from build123d import *

# Parameters (mm, degrees)
F0_W     = 127
F0_H     = 127
F1_DEPTH = 12.7
F3_D     = 15.24
F3_DEPTH = 12.7
F5_D     = 6.35
F5_DEPTH = 12.7


with BuildPart() as f1:
    # F0 (on Top) → F1 (new body)
    with BuildSketch(Plane.XY):
        with Locations((10.277962, -0.006821)):
            Rectangle(F0_W, F0_H)
    extrude(amount=F1_DEPTH)

    # F3
    with Locations(Plane.XY.offset(12.7)):
        with Locations((-40.522038, 50.793179), (-40.522038, 0), (-40.522038, -50.806821)):
            Hole(F3_D / 2, depth=F3_DEPTH)

    # F5
    with Locations(Plane.XY.offset(12.7)):
        with Locations((64.830244, -38.106821), (64.830244, 50.793179), (64.830244, 38.093179), (64.830244, -50.806821)):
            Hole(F5_D / 2, depth=F5_DEPTH)


solid = f1.part
Model file for the job. Use its own axes, mm. Give positions to 0.01 mm unless a question says otherwise; leave off trailing zeros. Loops run counter-clockwise (first coordinate to the right, second up) from the corner with the lowest first, then second, coordinate; pieces in that order, holes last.
Item 1: Drop a flat-ended pin along its axis: P1, Ø9, axis at x = -40.52, y = 50.79, coming from the -Z side. Give the stop position or say it passes through.
Check values:
P1: passes through
Item 2: Slice it at A-A (y = 0). Write the cut outline in (x, z), plus the area to 3 significant figures.
Check values:
outline: (-53.22, 0) - (-48.14, 0) - (-48.14, 12.7) - (-53.22, 12.7) - close; (-32.9, 0) - (73.78, 0) - (73.78, 12.7) - (-32.9, 12.7) - close
area: 1,420 mm2
Item 3: Slice it at B-B (z = 5.5). Write the cut outline in (x, y) (3 decimals).
Check values:
outline: (-53.222, -63.507) - (73.778, -63.507) - (73.778, 63.493) - (-53.222, 63.493) - close; hole circle Ø15.24 at (-40.522, -50.807); hole circle Ø15.24 at (-40.522, 0); hole circle Ø15.24 at (-40.522, 50.793); hole circle Ø6.35 at (64.83, -50.807); hole circle Ø6.35 at (64.83, -38.107); hole circle Ø6.35 at (64.83, 38.093); hole circle Ø6.35 at (64.83, 50.793)
Item 4: Mould opens along X. For faces 1 (the face through (9, 1, 0)), 2 (the face through (65.24, 53.94, 6.26)), 3 (the face through (73.778, -1, 6)) say: +X half, -X half, draft (parallel to the pull), parting line (faces both ways), or undercut.
Check values:
face 1: draft
face 2: undercut
face 3: +X half
Item 5: Drill centre lines: line 1 along X through (y, z) = (-48.5, 1.5); line 2 along X through (y, z) = (-0.5, 3); line 3 along X through (y, z) = (38, 8). Where is each one in solid material? Low to high.
Check values:
line 1: x = -53.22 to -47.78, -33.26 to 62.65, 67.01 to 73.78
line 2: x = -53.22 to -48.13, -32.92 to 73.78
line 3: x = -53.22 to 61.66, 68 to 73.78
